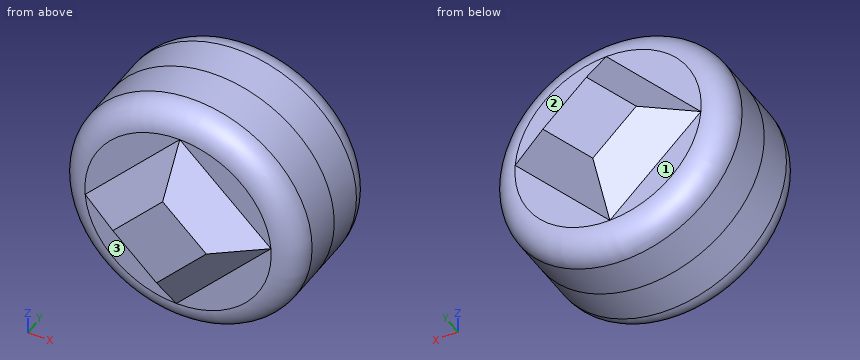
from build123d import *

# Parameters (mm, degrees)
F0_R     = 23.1993727041
F1_DEPTH = 12.7
F2_R     = 23.1993727041
F3_DEPTH = 12.7
F4_R     = 5.08
F7_DEPTH = 6.35
F8_DEPTH = 6.35
F9_SIZE  = 6.34999
F10_SIZE = 6.34999


# Not quite as in the source:
# - a fillet or chamfer is up to 0.001 mm smaller than in the source, because OpenCascade refuses the exact size


with BuildPart() as f1:
    # F0 (on Front) → F1 (new body)
    with BuildSketch(Plane.XZ):
        with Locations((-16.9251933694, -16.9251933694)):
            Circle(F0_R)
    extrude(amount=F1_DEPTH)

    # F2 (on face) → F3 (join)
    with BuildSketch(Plane(origin=(0, 0, 0), x_dir=(-1, 0, 0), z_dir=(0, 1, 0))):
        with Locations((16.9251933694, -16.9251933694)):
            Circle(F2_R)
    extrude(amount=F3_DEPTH)

    # F4
    f4_edges = [f1.edges().sort_by_distance(p)[0] for p in [
        (6.274179, 12.7, -16.925193),
        (-16.925193, 0, 6.274179),
        (-16.925193, 0, -40.124566),
        (6.274179, -6.35, -16.925193),
        (-40.124566, -12.7, -16.925193),
        (-40.124566, 6.35, -16.925193),
    ]]
    fillet(f4_edges, radius=F4_R)

    # F5 (on face) → F7 (join)
    with BuildSketch(Plane(origin=(0, 12.7, 0), x_dir=(-1, 0, 0), z_dir=(0, 1, 0))):
        Polygon((34.987336153, -18.3641740003), (16.5690030176, 1.1906780042), (-1.1369494142, -15.4862127385), (17.2813837212, -35.041064743), align=None)
    extrude(amount=F7_DEPTH)

    # F6 (on face) → F8 (join)
    with BuildSketch(Plane.XZ.offset(12.7)):
        Polygon((1.1413726115, -15.5428544637), (-16.5892601531, 1.1910649658), (-34.9917593503, -18.3075322751), (-17.2611265857, -35.0414517045), align=None)
    extrude(amount=F8_DEPTH)

    # F9 (size 6.35 in the source; OpenCascade refuses exactly that, so slightly less here)
    f9_edges = [f1.edges().sort_by_distance(p)[0] for p in [
        (-8.072217, 19.05, -25.263639),
        (-26.13436, 19.05, -26.702619),
        (-25.77817, 19.05, -8.586748),
        (-7.716027, 19.05, -7.147767),
    ]]
    chamfer(f9_edges, length=F9_SIZE)

    # F10 (size 6.35 in the source; OpenCascade refuses exactly that, so slightly less here)
    f10_edges = [f1.edges().sort_by_distance(p)[0] for p in [
        (-8.059877, -19.05, -25.292153),
        (-7.723944, -19.05, -7.175895),
        (-25.79051, -19.05, -8.558234),
        (-26.126443, -19.05, -26.674492),
    ]]
    chamfer(f10_edges, length=F10_SIZE)


solid = f1.part
Check sheet for the modelled part. Datum: model origin and axes. Units: mm. Face numbers are marked on the shaded views. A direction names the side the tool comes from. Coordinates: 2 decimals unless noted, no trailing zeros. Write each loop counter-clockwise with the first axis right and the second up, starting at its lowest first coordinate (ties: lowest second). Pieces come first, ordered by that corner, then holes. Notation, with made-up numbers: M 40,78 L 64,78 A26 cw 64,115 Z; hole C 54,-10 d6. An arc over 180 degrees is marked long. Answer as CSV lines item,"result".
Q1. Cross-section at D-D (y = 1). Record the boundary of the cut face in (x, z), then the cut area to 3 significant figures.
Check result:
outline,"C -16.93,-16.93 d46.4"
area,"1,690 mm^2"
Q2. Cross-section at A-A (y = 9.5). Record the boundary of the cut face in (x, z).
Check result:
outline,"C -16.93,-16.93 d45.68"
Q3. Cross-section at C-C (y = 15). Record the boundary of the cut face in (x, z).
Check result:
outline,"M -31.74,-18.27 L -17.38,-31.79 L -2.11,-15.58 L -16.47,-2.06 Z"
Q4. Set-up check for the marked faces 1, 2 and 3: record each of +Z, -Z, +X, -X, +Y, -Y from which the full face is reachable in a straight line by a thin tool's end or side.
Check result:
face 1,"-Z, -X, +Y"
face 2,"+Z, +X, +Y"
face 3,"-Z, -X, -Y"
Q5. Go/stop test with flat-tipped pins: pin 1 (13.5 mm diameter, centred on x = -30, z = -24.5, fed in from +Y); pin 2 (5 mm diameter, centred on y = -13.5, z = -30.5, fed in from +X); pin 3 (20.5 mm diameter, centred on x = -26, z = -4, fed in from +Y); pin 4 (5 mm diameter, centred on x = -5.5, z = -5.5, fed in from +Y). Record where each tip stops, or that it passes through.
Check result:
pin 1,"y = 18.4"
pin 2,"x = 0.8"
pin 3,"y = 19.05"
pin 4,"y = 12.7"
Q6. Material ranges on probe 1 along Y at (x, z) = (-5, -22.5); probe 2 along X at (y, z) = (-2.5, -30); probe 3 along X at (y, z) = (3, -29), recorded low to high. Write a range as from..to.
Check result:
probe 1,"-12.7..12.7"
probe 2,"-36.09..2.24"
probe 3,"-36.73..2.88"
Q7. Cross-section at B-B (y = -14.5). Record the boundary of the cut face in (x, z), then the cut area to 3 significant figures.
Check result:
outline,"M -32.45,-18.23 L -17.33,-32.5 L -1.4,-15.62 L -16.52,-1.35 Z"
area,"482 mm^2"
